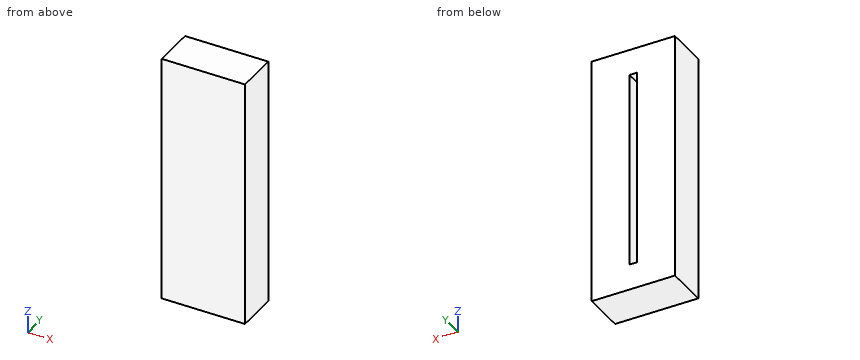
from build123d import *

# Parameters (mm, degrees)
SKETCH1_W           = 101.6
SKETCH1_H           = 50.8
BOSS_EXTRUDE1_DEPTH = 304.8
CUT_EXTRUDE1_DEPTH  = 19.05


with BuildPart() as part:
    # Sketch1 → Boss-Extrude1 (new body)
    with BuildSketch(Plane.XY):
        with Locations((50.8, 25.4)):
            Rectangle(SKETCH1_W, SKETCH1_H)
    extrude(amount=BOSS_EXTRUDE1_DEPTH)

    # Sketch2 → Cut-Extrude1 (cut)
    with BuildSketch(Plane(origin=(0, 50.8, 0), x_dir=(1, 0, 0), z_dir=(0, 1, 0))):
        Polygon((46.0375, -41.275), (46.0375, -31.75), (55.5625, -31.75), (55.5625, -41.275), (55.5625, -263.525), (55.5625, -273.05), (46.0375, -273.05), (46.0375, -263.525), align=None)
    extrude(amount=-CUT_EXTRUDE1_DEPTH, mode=Mode.SUBTRACT)


solid = part.part
The listing builds one solid part. Answer for the finished solid, in the listing's coordinates (mm). Give positions to 0.01 mm unless a question says otherwise; leave off trailing zeros. Loops run counter-clockwise (first coordinate to the right, second up) from the corner with the lowest first, then second, coordinate; pieces in that order, holes last.
Item 1: Find the intervals of material crossed by line 1 along X through (y, z) = (41, 102.5); line 2 along Z through (x, y) = (50.5, 44); line 3 along Y through (x, z) = (50.5, 129.5), in increasing order.
Derived:
line 1: x = 0 to 46.04, 55.56 to 101.6
line 2: z = 0 to 31.75, 273.05 to 304.8
line 3: y = 0 to 31.75
Item 2: A cutting plane is placed at B-B (z = 114). Give the vertices of the cut face in (x, y), then the cut area to 3 significant figures.
Derived:
outline: (0, 0) - (101.6, 0) - (101.6, 50.8) - (55.56, 50.8) - (55.56, 31.75) - (46.04, 31.75) - (46.04, 50.8) - (0, 50.8) - close
area: 4,980 mm2
Item 3: A cutting plane is placed at A-A (y = 38). Give the vertices of the cut face in (x, z), then the cut area to 3 significant figures.
Derived:
outline: (0, 0) - (101.6, 0) - (101.6, 304.8) - (0, 304.8) - close; hole (46.04, 31.75) - (55.56, 31.75) - (55.56, 273.05) - (46.04, 273.05) - close
area: 28,700 mm2
